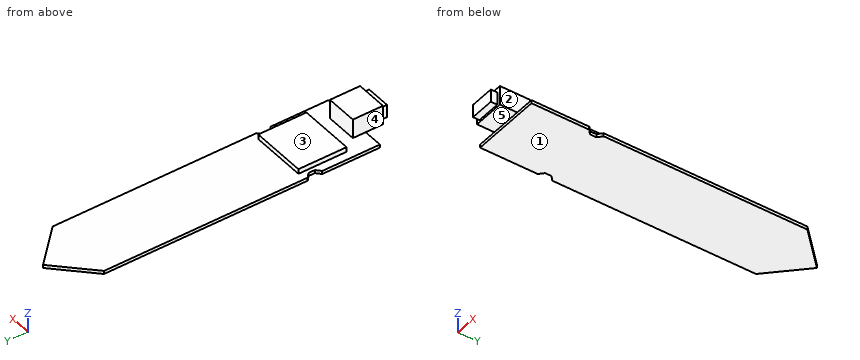
Autodesk Inventor part; units mm, degrees
ref_plane "YZ Plane" through (0, 0, 0) normal (1, 0, 0) x (0, 1, 0)
ref_plane "XZ Plane" through (0, 0, 0) normal (0, 1, 0) x (-1, 0, 0)
ref_plane "XY Plane" through (0, 0, 0) normal (0, 0, 1) x (1, 0, 0)
sketch "Skizze1" plane through (0, 0, 0) normal (0, 0, 1) x (1, 0, 0)
  line L0 (11, -43) -> (-11, -43)
  line L1 (-11, -43) -> (-11, 43)
  line L2 (11, 43) -> (11, -43)
  line L3 (11, -43) -> (-11, 43) construction
  line L4 (-11, -43) -> (11, 43) construction
  line L5 (-11, 43) -> (0, 54)
  line L6 (0, 54) -> (11, 43)
  point P0 (0, 0)
  point P1 (0, 0)
  dimension "d0" = 22
  dimension "d1" = 86
  dimension "d2" = 97
extrude "Extrusion1" add sketch "Skizze1" along normal mid plane 1
sketch "Skizze2" plane through (0, 0, 0.5) normal (0, 0, 1) x (1, 0, 0)
  line L0 (-11, -20.5) -> (-9.6, -21.75)
  line L1 (-9.6, -21.75) -> (-9.6, -23.75)
  line L2 (-9.6, -23.75) -> (-11, -25)
  line L3 (-11, -25) -> (-11, -20.5)
  line L4 (-11, 43) -> (-11, -43)
  point P0 (0, 0)
  point P1 (-11, -22.75)
  point P2 (-9.6, -22.75)
  dimension "d5" = 1.4
  dimension "d6" = 18
  dimension "d7" = 22.5
  dimension "d8" = 2
extrude "Extrusion2" cut sketch "Skizze2" against normal blind 1
mirror "Spiegeln1" about plane through (0, 0, 0) normal (1, 0, 0) of "Extrusion2"
sketch "Skizze3" plane through (0, 0, 0.5) normal (0, 0, 1) x (1, 0, 0)
  line L0 (-4.9, -39) -> (4.9, -39)
  line L1 (4.9, -39) -> (4.9, -48.4)
  line L2 (4.9, -48.4) -> (-4.9, -48.4)
  line L3 (-4.9, -48.4) -> (-4.9, -39)
  line L4 (-11, -43) -> (11, -43)
  point P0 (0, 0)
  point P1 (0, -39)
  point P2 (0, -43)
  dimension "d11" = 9.4
  dimension "d12" = 9.8
  dimension "d13" = 5.4
extrude "Extrusion3" add sketch "Skizze3" along normal blind 6
sketch "Skizze4" plane through (0, 0, 0.5) normal (0, 0, 1) x (1, 0, 0)
  line L0 (-8.4, -19.5) -> (8.8, -19.5)
  line L1 (8.8, -19.5) -> (8.8, -34.5)
  line L2 (8.8, -34.5) -> (-8.4, -34.5)
  line L3 (-8.4, -34.5) -> (-8.4, -19.5)
  line L4 (4.9, -43) -> (11, -43)
  line L5 (11, -43) -> (11, -25)
  line L6 (-11, -25) -> (-11, -43)
  point P0 (0, 0)
  dimension "d16" = 23.5
  dimension "d19" = 8.5
  dimension "d20" = 2.2
  dimension "d21" = 2.6
extrude "Extrusion4" add sketch "Skizze4" along normal blind 1.5
sketch "Skizze5" plane through (-4.9, -48.4, 0.5) normal (0, -1, 0) x (1, 0, 0)
  line L0 (1.0328, 4.6703) -> (8.6704, 4.6703)
  line L1 (8.6704, 4.6703) -> (8.6704, 0.6911)
  line L2 (8.6704, 0.6911) -> (1.0328, 0.6911)
  line L3 (1.0328, 0.6911) -> (1.0328, 4.6703)
  point P0 (4.9, -0.5)
extrude "Extrusion5" add sketch "Skizze5" along normal blind 2
properties part number "CSM_Sensor_Dummy"
Could you check a few things on this model? Use its own coordinates, in mm. Face numbers are marked on the shaded views. A direction names the side the tool comes from. Give positions to 0.01 mm unless a question says otherwise; leave off trailing zeros. Order: outer loops, then holes, each group sorted by start corner. A loop starts at its lowest first (then second) coordinate and runs counter-clockwise, first axis right, second up. Notation, with made-up numbers: (3.5, 40.5) -> (48.5, 40.5) arc R26 cw to (48.5, 67.5) -> close; hole circle Ø9 at (21.25, -27). An arc over 180 degrees is marked (long way). Return JSON: item names as keys, results as strings.
1. Imagine slicing it at D-D on y = 4. List the corners of the cut face in (x, z) for me, then the cut area to 3 significant figures.
Answer list:
{"outline": "(-11, -0.5) -> (11, -0.5) -> (11, 0.5) -> (-11, 0.5) -> close", "area": "22.0 mm2"}
2. I need wall thicknesses on line 1 (Y direction, x = 4.5, z = 6.25); line 2 (Z direction, x = -3.5, y = 25.5); line 3 (Y direction, x = 1, z = 3). Which ranges of each line are inside material? Lowest first, please. Write a range as from..to.
Answer list:
{"line 1": "y = -48.4..-39", "line 2": "z = -0.5..0.5", "line 3": "y = -50.4..-39"}
3. Imagine slicing it at A-A on z = 3. List the corners of the cut face in (x, y) for me, then the cut area to 3 significant figures.
Answer list:
{"outline": "(-4.9, -48.4) -> (-3.87, -48.4) -> (-3.87, -50.4) -> (3.77, -50.4) -> (3.77, -48.4) -> (4.9, -48.4) -> (4.9, -39) -> (-4.9, -39) -> close", "area": "107 mm2"}
4. For pin 1 Ø2 at (x, y) = (-7, -39.5) entering from +Z; pin 2 Ø4 at (x, z) = (-7.5, 3) entering from -Y; pin 3 Ø0.8 at (y, z) = (-25, 1.5) entering from +X, each with a flat end and sliding along its axis, tell me the tip position at first contact or that it passes through.
Answer list:
{"pin 1": "stops at z = 0.5", "pin 2": "stops at y = -34.5", "pin 3": "stops at x = 8.8"}
5. Imagine slicing it at B-B on x = 7.25. List the corners of the cut face in (y, z) for me.
Answer list:
{"outline": "(-43, -0.5) -> (46.75, -0.5) -> (46.75, 0.5) -> (-19.5, 0.5) -> (-19.5, 2) -> (-34.5, 2) -> (-34.5, 0.5) -> (-43, 0.5) -> close"}
6. Imagine slicing it at C-C on y = -44. List the corners of the cut face in (x, z) for me.
Answer list:
{"outline": "(-4.9, 0.5) -> (4.9, 0.5) -> (4.9, 6.5) -> (-4.9, 6.5) -> close"}
7. On a 3-axis mill with a long thin cutter (end or side, diameter ignored), from which of +Z, -Z, +X, -X, +Y, -Y can I reach the whole of each face in a straight line? I mean the marked faces 1, 2, 3, 4 and 5. Say none if no direction works.
Answer list:
{"face 1": "-Z, +X, -X, +Y, -Y", "face 2": "+Z, +X, -Y", "face 3": "+Z, +X, -X, +Y", "face 4": "+Z, -X, -Y", "face 5": "-Z, +X, -X, -Y"}
